Geometry: final body of the model. Coordinates: model frame, mm. Give positions to 0.01 mm unless a question says otherwise; leave off trailing zeros. Loops run counter-clockwise (first coordinate to the right, second up) from the corner with the lowest first, then second, coordinate; pieces in that order, holes last.
1. Section A-A, the plane z = -2.5. Output: boundary loops of the cut face in (x, y).
2. Section C-C, the plane y = 8.5. Output: boundary loops of the cut face in (x, z).
3. Section B-B, the plane x = 0.5. Output: boundary loops of the cut face in (y, z).
4. First-contact query: P1, Ø0.9, axis at x = 1.5, y = 15.5, coming from the -Z side; P2, Ø0.9, axis at x = 2, z = 8, coming from the +Y side; P3, Ø1.5, axis at x = 2, y = 6.5, coming from the +Z side. Flat tips, straight axial feed; report the tip coordinate or a pass-through.
5. Material intervals for line 1 along Z through (x, y) = (1.45, -22); line 2 along Y through (x, z) = (1.6, 5.75); line 3 along Y through (x, z) = (1.4, 5), sorted ascending.
from build123d import *

# Parameters (mm, degrees)
F1_DEPTH = 3


with BuildPart() as f1:
    # F0 (on Right) → F1 (new body)
    with BuildSketch(Plane.YZ):
        with BuildLine():
            Line((-34.952577, -0.875086), (0, -0.875086))
            Line((0, -0.875086), (34.952577, -0.875086))
            ThreePointArc((34.952577, -0.875086), (36.32333, -2.245839), (34.952577, -3.616591))
            ThreePointArc((34.952577, -3.616591), (43.813866, 0.767528), (39.71675, 9.765116))
            Line((39.71675, 9.765116), (37.631799, 9.765116))
            Line((37.631799, 9.765116), (38.35, 9.040914))
            Line((38.35, 9.040914), (38.35, 7.190914))
            ThreePointArc((38.35, 7.190914), (36.270899, 6.728344), (35.65, 4.690914))
            Line((35.65, 4.690914), (0, 4.690914))
            Line((0, 4.690914), (-35.65, 4.690914))
            ThreePointArc((-35.65, 4.690914), (-36.270899, 6.728344), (-38.35, 7.190914))
            Line((-38.35, 7.190914), (-38.35, 9.040914))
            Line((-38.35, 9.040914), (-37.631799, 9.765116))
            Line((-37.631799, 9.765116), (-39.71675, 9.765116))
            ThreePointArc((-39.71675, 9.765116), (-43.813866, 0.767528), (-34.952577, -3.616591))
            ThreePointArc((-34.952577, -3.616591), (-36.32333, -2.245839), (-34.952577, -0.875086))
        make_face()
    extrude(amount=F1_DEPTH)


solid = f1.part
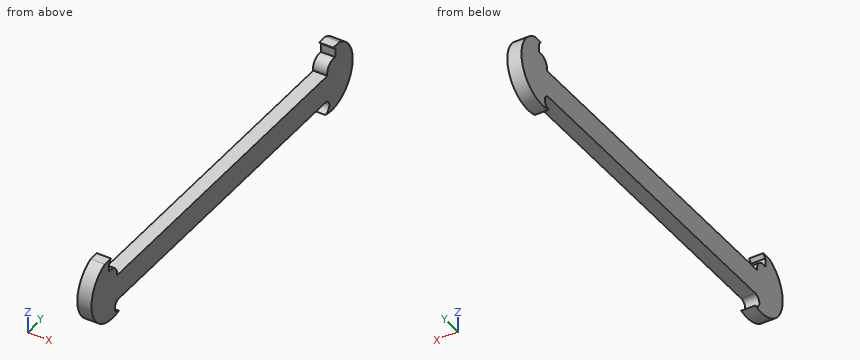
Answers below:
1. outline: (0, -41.43) - (3, -41.43) - (3, -36.3) - (0, -36.3) - close; (0, 36.3) - (3, 36.3) - (3, 41.43) - (0, 41.43) - close
2. outline: (0, -0.88) - (3, -0.88) - (3, 4.69) - (0, 4.69) - close
3. outline: (-39.72, 9.77) arc R7.11 ccw to (-34.95, -3.62) arc R1.37 cw to (-34.95, -0.88) - (34.95, -0.88) arc R1.37 cw to (34.95, -3.62) arc R7.11 ccw to (39.72, 9.77) - (37.63, 9.77) - (38.35, 9.04) - (38.35, 7.19) arc R2.11 ccw to (35.65, 4.69) - (-35.65, 4.69) arc R2.11 ccw to (-38.35, 7.19) - (-38.35, 9.04) - (-37.63, 9.77) - close
4. P1: stops at z = -0.88
4. P2: stops at y = 42.7
4. P3: stops at z = 4.69
5. line 1: z = -0.88 to 4.69
5. line 2: y = -43.73 to -35.67, 35.67 to 43.73
5. line 3: y = -43.98 to -35.6, 35.6 to 43.98
